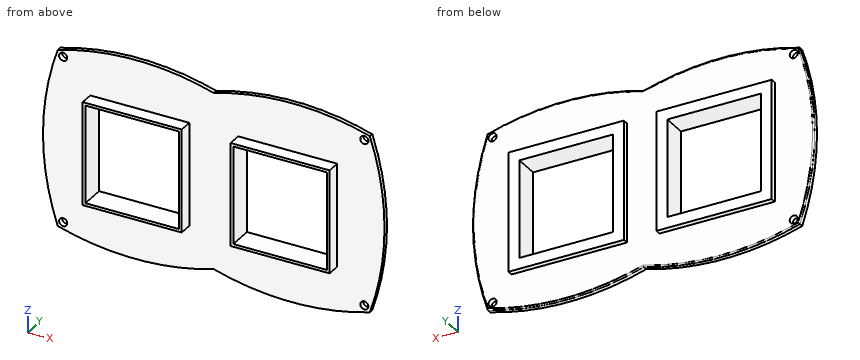
from build123d import *

# Parameters (mm, degrees)
BOSS_EXTRUDE1_DEPTH = 2
HOLE1_D             = 3
HOLE1_DEPTH         = 10
FILLET1_R           = 0.5
SKETCH7_W           = 34.5
SKETCH7_H           = 36
CUT_EXTRUDE1_DEPTH  = 2
SKETCH9_W           = 36.5
SKETCH9_H           = 38
SKETCH9_W_2         = 34.5
SKETCH9_H_2         = 36
BOSS_EXTRUDE2_DEPTH = 5
SKETCH10_W          = 42.5
SKETCH10_H          = 44
SKETCH10_W_2        = 34.5
SKETCH10_H_2        = 36
BOSS_EXTRUDE3_DEPTH = 2


with BuildPart() as part:
    # Sketch2 → Boss-Extrude1 (new body)
    with BuildSketch(Plane(origin=(0, 0, 0), x_dir=(1, 0, 0), z_dir=(0, 1, 0))):
        with BuildLine():
            ThreePointArc((-57.5, 32.5), (-28.75, 36.721936228), (0, 32.5))
            ThreePointArc((0, 32.5), (28.75, 36.721936228), (57.5, 32.5))
            ThreePointArc((57.5, 32.5), (62.928598403, 0), (57.5, -32.5))
            ThreePointArc((57.5, -32.5), (28.75, -36.721936228), (0, -32.5))
            ThreePointArc((0, -32.5), (-28.75, -36.721936228), (-57.5, -32.5))
            ThreePointArc((-57.5, -32.5), (-62.928598403, 0), (-57.5, 32.5))
        make_face()
    extrude(amount=BOSS_EXTRUDE1_DEPTH)

    # Hole1
    with Locations(Plane(origin=(0, 2, 0), x_dir=(1, 0, 0), z_dir=(0, 1, 0))):
        with Locations((-55.5, 30.5), (55.5, 30.5), (55.5, -30.5), (-55.5, -30.5)):
            Hole(HOLE1_D / 2, depth=HOLE1_DEPTH)

    # Fillet1
    fillet1_edges = [part.edges().sort_by_distance(p)[0] for p in [
        (28.75, 2, 36.721936228),
        (62.928598403, 2, 0),
        (28.75, 2, -36.721936228),
        (-28.75, 2, -36.721936228),
        (-62.928598403, 2, 0),
        (-28.75, 2, 36.721936228),
    ]]
    fillet(fillet1_edges, radius=FILLET1_R)

    # Sketch7 → Cut-Extrude1 (cut)
    with BuildSketch(Plane(origin=(0, 2, 0), x_dir=(1, 0, 0), z_dir=(0, 1, 0))):
        with Locations((-27.25, 0)):
            Rectangle(SKETCH7_W, SKETCH7_H)
    cut_extrude1 = extrude(amount=-CUT_EXTRUDE1_DEPTH, mode=Mode.SUBTRACT)

    # Sketch9 → Boss-Extrude2 (add)
    with BuildSketch(Plane.XZ):
        with Locations((-27.25, 0)):
            Rectangle(SKETCH9_W, SKETCH9_H)
        with Locations((-27.25, 0)):
            Rectangle(SKETCH9_W_2, SKETCH9_H_2, mode=Mode.SUBTRACT)
    boss_extrude2 = extrude(amount=BOSS_EXTRUDE2_DEPTH)

    # Sketch10 → Boss-Extrude3 (add)
    with BuildSketch(Plane(origin=(0, 2, 0), x_dir=(1, 0, 0), z_dir=(0, 1, 0))):
        with Locations((-27.25, 0)):
            Rectangle(SKETCH10_W, SKETCH10_H)
        with Locations((-27.25, 0)):
            Rectangle(SKETCH10_W_2, SKETCH10_H_2, mode=Mode.SUBTRACT)
    boss_extrude3 = extrude(amount=BOSS_EXTRUDE3_DEPTH)

    # Mirror1: Cut-Extrude1, Boss-Extrude2, Boss-Extrude3 across plane
    add(cut_extrude1.mirror(Plane(origin=(0, 0, 0), x_dir=(0, 0, 1), z_dir=(1, 0, 0))), mode=Mode.SUBTRACT)
    add(boss_extrude2.mirror(Plane(origin=(0, 0, 0), x_dir=(0, 0, 1), z_dir=(1, 0, 0))))
    add(boss_extrude3.mirror(Plane(origin=(0, 0, 0), x_dir=(0, 0, 1), z_dir=(1, 0, 0))))


solid = part.part
Can you work these out from the model? Positions are in its coordinate system, mm. Give positions to 0.01 mm unless a question says otherwise; leave off trailing zeros. Order: outer loops, then holes, each group sorted by start corner. A loop starts at its lowest first (then second) coordinate and runs counter-clockwise, first axis right, second up. Notation, with made-up numbers: M 75,63.5 L 101,63.5 A19 cw 101,75.5 Z; hole C -12.5,70.5 d3. An arc over 180 degrees is marked long. Use a Markdown table: item, result. Add a question column.
Item 1: Suppose I cut it at A-A (y = -1.25). List the corners of the cut face in (x, z) for me, then the cut area to 3 significant figures.
Item 2: Will these pins go through, and if not, where does the flat tip stop? pin 1 (1 mm diameter, centred on x = -35.5, y = 3, fed in from -Z); pin 2 (2.5 mm diameter, centred on y = -1.5, z = -4, fed in from -X); pin 3 (1 mm diameter, centred on x = 42, z = -24.5, fed in from -Y).
Item 3: Suppose I cut it at B-B (z = 4). Count the separate pieces of the cut face and the enclosed holes in it, then the cut area to 3 significant figures.
Item 4: If I drill on L1, parallel to X at y = -2.75, z = 12; L2, parallel to Z at x = 21, y = -3.5; L3, parallel to Z at x = 55.5, y = 1.3, over which ranges is the centre line in solid material (lowest first)? Write a range as [from, to].
Answer sheet:
| question | item | result |
|---|---|---|
| 1 | outline | M -45.5,-19 L -9,-19 L -9,19 L -45.5,19 Z; M 9,-19 L 45.5,-19 L 45.5,19 L 9,19 Z; hole M -44.5,-18 L -10,-18 L -10,18 L -44.5,18 Z; hole M 10,-18 L 44.5,-18 L 44.5,18 L 10,18 Z |
| 1 | area | 290 mm² |
| 2 | pin 1 | stops at z = -22 |
| 2 | pin 2 | stops at x = -45.5 |
| 2 | pin 3 | stops at y = 0 |
| 3 | separate pieces | 3 |
| 3 | enclosed holes | 0 |
| 3 | area | 165 mm² |
| 4 | L1 | x = [-45.5, -44.5], [-10, -9], [9, 10], [44.5, 45.5] |
| 4 | L2 | z = [-19, -18], [18, 19] |
| 4 | L3 | z = [-33.08, -32], [-29, 29], [32, 33.08] |
